Design review of the part built by this model. Coordinates are the model's own, in mm. A direction names the side the tool comes from. Give positions to 0.01 mm unless a question says otherwise; leave off trailing zeros. Write each loop counter-clockwise with the first axis right and the second up, starting at its lowest first coordinate (ties: lowest second). Pieces come first, ordered by that corner, then holes. Notation, with made-up numbers: (17.25, 29) -> (70.25, 29) arc R19 ccw to (70.25, 38) -> close; hole circle Ø1 at (-14.75, 82). An arc over 180 degrees is marked (long way). Return JSON: item names as keys, results as strings. Group by question number.
from build123d import *

# Parameters (mm, degrees)
BOSS_EXTRUDE1_DEPTH      = 15
BOSS_EXTRUDE1_DEPTH_BACK = 15
SKETCH1_W                = 45
SKETCH1_H                = 40
CUT_EXTRUDE1_DEPTH       = 12.75
CUT_EXTRUDE1_DEPTH_BACK  = 12.75
SKETCH2_W                = 38
SKETCH2_H                = 15
FILLET1_R                = 13
FILLET2_R                = 2


with BuildPart() as part:
    # Sketch1 → Boss-Extrude1 (new, two sides: drawn at the far end of the back side and taken through both)
    with BuildSketch(Plane(origin=(0, 0, 0), x_dir=(1, 0, 0), z_dir=(0, 1, 0)).offset(-BOSS_EXTRUDE1_DEPTH_BACK)):
        Rectangle(SKETCH1_W, SKETCH1_H)
    extrude(amount=BOSS_EXTRUDE1_DEPTH + BOSS_EXTRUDE1_DEPTH_BACK)

    # Sketch2 → Cut-Extrude1 (cut, two sides: drawn at the far end of the back side and taken through both)
    with BuildSketch(Plane(origin=(0, 0, 0), x_dir=(1, 0, 0), z_dir=(0, 1, 0)).offset(-CUT_EXTRUDE1_DEPTH_BACK)):
        with Locations((3.5, 10)):
            Rectangle(SKETCH2_W, SKETCH2_H)
        with Locations((3.5, -10)):
            Rectangle(SKETCH2_W, SKETCH2_H)
    extrude(amount=CUT_EXTRUDE1_DEPTH + CUT_EXTRUDE1_DEPTH_BACK, mode=Mode.SUBTRACT)

    # Fillet1
    # the kernel refuses this fillet: 13 mm, written as the material it adds along each edge
    with BuildSketch(Plane(origin=(-15.5, -12.75, -17.5), x_dir=(1, 0, 0), z_dir=(0, 0, 1))) as fillet1_piece_1_section:
        with BuildLine():
            CenterArc((FILLET1_R, FILLET1_R), FILLET1_R, 180, 90)
            Line((0, FILLET1_R), (0, 0))
            Line((0, 0), (FILLET1_R, 0))
        make_face()
    fillet1_piece_1 = extrude(amount=47.5, mode=Mode.PRIVATE)
    fillet1_piece_1 = split(fillet1_piece_1, bisect_by=Plane(origin=(-12.596216794, -9.846216794, 17.5), z_dir=(0, 0, -1)), keep=Keep.TOP, mode=Mode.PRIVATE)
    add(fillet1_piece_1)
    with BuildSketch(Plane(origin=(-15.5, 12.75, -17.5), x_dir=(1, 0, 0), z_dir=(0, 0, 1))) as fillet1_piece_2_section:
        with BuildLine():
            CenterArc((FILLET1_R, -FILLET1_R), FILLET1_R, 90, 90)
            Line((0, -FILLET1_R), (0, 0))
            Line((0, 0), (FILLET1_R, 0))
        make_face()
    fillet1_piece_2 = extrude(amount=47.5, mode=Mode.PRIVATE)
    fillet1_piece_2 = split(fillet1_piece_2, bisect_by=Plane(origin=(-12.596216794, 9.846216794, 17.5), z_dir=(0, 0, -1)), keep=Keep.TOP, mode=Mode.PRIVATE)
    add(fillet1_piece_2)
    with BuildSketch(Plane(origin=(-15.5, 12.75, 17.5), x_dir=(1, 0, 0), z_dir=(0, 0, -1))) as fillet1_piece_3_section:
        with BuildLine():
            CenterArc((FILLET1_R, FILLET1_R), FILLET1_R, 180, 90)
            Line((0, FILLET1_R), (0, 0))
            Line((0, 0), (FILLET1_R, 0))
        make_face()
    fillet1_piece_3 = extrude(amount=47.5, mode=Mode.PRIVATE)
    fillet1_piece_3 = split(fillet1_piece_3, bisect_by=Plane(origin=(-12.596216794, 9.846216794, -17.5), z_dir=(0, 0, 1)), keep=Keep.TOP, mode=Mode.PRIVATE)
    add(fillet1_piece_3)
    with BuildSketch(Plane(origin=(-15.5, -12.75, 17.5), x_dir=(1, 0, 0), z_dir=(0, 0, -1))) as fillet1_piece_4_section:
        with BuildLine():
            CenterArc((FILLET1_R, -FILLET1_R), FILLET1_R, 90, 90)
            Line((0, -FILLET1_R), (0, 0))
            Line((0, 0), (FILLET1_R, 0))
        make_face()
    fillet1_piece_4 = extrude(amount=47.5, mode=Mode.PRIVATE)
    fillet1_piece_4 = split(fillet1_piece_4, bisect_by=Plane(origin=(-12.596216794, -9.846216794, -17.5), z_dir=(0, 0, 1)), keep=Keep.TOP, mode=Mode.PRIVATE)
    add(fillet1_piece_4)

    # Fillet2
    fillet2_edges = [part.edges().sort_by_distance(p)[0] for p in [
        (0, 15, -20),
        (-22.5, 15, 0),
        (0, 15, 20),
        (0, -15, -20),
        (22.5, 15, 0),
        (-22.5, -15, 0),
        (0, -15, 20),
        (-22.5, 0, 20),
        (-22.5, 0, -20),
        (22.5, 0, -20),
        (22.5, 0, 20),
        (22.5, -15, 0),
    ]]
    fillet(fillet2_edges, radius=FILLET2_R)

    # Sketch3 → Revolve1 (revolve)
    with BuildSketch(Plane(origin=(0, 0, 0), x_dir=(1, 0, 0), z_dir=(0, 1, 0))):
        Polygon((-22.5, 0), (-32.5, 0), (-22.5, 5), align=None)
    revolve(axis=Axis((-22.5, 0, 0), (-1, 0, 0)))


solid = part.part
Q1. Take a section at A-A, the plane x = 10. Give the boundary of the cut face in (y, z).
Q2. For L1, parallel to Z at x = 17, y = 10.5; L2, parallel to Y at x = 2, z = -5.5; L3, parallel to X at y = 5, z = 1.5, list the stretches that pass through material, from the lowest coordinate up. Write a range as from..to.
Q3. Insertion check: pin 1 (4 mm diameter, centred on y = 4.5, z = 13.5, fed in from -X); pin 2 (1 mm diameter, centred on y = -7.5, z = 4.5, fed in from +X). Each pin has a flat end and moves straight along its axis. Give the tip position at first contact, or say it passes through.
Q4. Take a section at B-B, the plane z = 7. Give the boundary of the cut face in (x, y).
Q5. Mouldability with a two-part tool opening along Z and no side actions: class faces 1 (the face through (0.29, -14.43, -19.4)), 2 (the face through (-22.5, -3.1, 4.3)), 3 (the face through (10, 12.75, 10)) as +Z half, -Z half, draft (parallel to the pull), parting line (faces both ways), or undercut.
Q6. Tool access review of faces 4 (the face through (3, 0, 17.5)), 5 (the face through (21.93, 14.4, -0.25)): name each direction out of +Z, -Z, +X, -X, +Y, -Y from which nothing blocks a thin tool from reaching the whole face with its end or side.
Q7. Take a section at C-C, the plane x = -11.5. Give the boundary of the cut face in (y, z).
Q8. Take a section at D-D, the plane x = -28. Give the boundary of the cut face in (y, z), plus the area to 3 significant figures.
Final values:
{
 "1": {"outline": "(-15, -18) arc R2 ccw to (-13, -20) -> (13, -20) arc R2 ccw to (15, -18) -> (15, 18) arc R2 ccw to (13, 20) -> (-13, 20) arc R2 ccw to (-15, 18) -> close; hole (-12.75, -17.5) -> (12.75, -17.5) -> (12.75, -2.5) -> (-12.75, -2.5) -> close; hole (-12.75, 2.5) -> (12.75, 2.5) -> (12.75, 17.5) -> (-12.75, 17.5) -> close"},
 "2": {"L1": "z = -20..-17.5, -2.5..2.5, 17.5..20", "L2": "y = -15..-12.75, 12.75..15", "L3": "x = -22.5..22.5"},
 "3": {"pin 1": "stops at x = -22.5", "pin 2": "stops at x = -12.55"},
 "4": {"outline": "(-22.5, -13) arc R2 ccw to (-20.5, -15) -> (20.5, -15) arc R2 ccw to (22.5, -13) -> (22.5, -12.75) -> (-2.5, -12.75) arc R13 cw to (-15.5, 0) arc R13 cw to (-2.5, 12.75) -> (22.5, 12.75) -> (22.5, 13) arc R2 ccw to (20.5, 15) -> (-20.5, 15) arc R2 ccw to (-22.5, 13) -> close"},
 "5": {"face 1": "-Z half", "face 2": "draft", "face 3": "undercut"},
 "6": {"face 4": "+X", "face 5": "+Z, -Z, +X, +Y"},
 "7": {"outline": "(-15, -18) arc R2 ccw to (-13, -20) -> (13, -20) arc R2 ccw to (15, -18) -> (15, 18) arc R2 ccw to (13, 20) -> (-13, 20) arc R2 ccw to (-15, 18) -> close; hole (-9.13, -17.5) -> (9.13, -17.5) -> (9.13, -2.5) -> (-9.13, -2.5) -> close; hole (-9.13, 2.5) -> (9.13, 2.5) -> (9.13, 17.5) -> (-9.13, 17.5) -> close"},
 "8": {"outline": "circle Ø4.5 at (0, 0)", "area": "15.9 mm²"}
}
